from build123d import *

# Parameters (mm, degrees)
BOSS_EXTRUDE1_DEPTH = 11
SKETCH3_W           = 22
SKETCH3_H           = 3
BOSS_EXTRUDE2_DEPTH = 10.2
BOSS_EXTRUDE3_DEPTH = 5
SKETCH5_R           = 1.035
SKETCH5_R_2         = 1.1
CUT_EXTRUDE1_DEPTH  = 34.004922045
SKETCH6_W           = 7
SKETCH6_H           = 7
BOSS_EXTRUDE4_DEPTH = 5
SKETCH7_R           = 1.65
CUT_EXTRUDE2_DEPTH  = 29.50349942
FILLET1_R           = 1


with BuildPart() as part:
    # Sketch1 → Boss-Extrude1 (new, symmetric)
    with BuildSketch(Plane(origin=(0, 0, 0), x_dir=(0, 0, -1), z_dir=(1, 0, 0))):
        Polygon((-13.0089, 0), (13.0089, 0), (13.0089, 3), (5.7589, 3), (5.7589, 1.5), (-5.7589, 1.5), (-5.7589, 3), (-13.0089, 3), align=None)
    extrude(amount=BOSS_EXTRUDE1_DEPTH, both=True)

    # Sketch3 → Boss-Extrude2 (add)
    with BuildSketch(Plane.XZ):
        with Locations((0, -14.5089)):
            Rectangle(SKETCH3_W, SKETCH3_H)
        with Locations((0, 14.5089)):
            Rectangle(SKETCH3_W, SKETCH3_H)
    extrude(amount=-BOSS_EXTRUDE2_DEPTH)

    # Sketch4 → Boss-Extrude3 (add)
    with BuildSketch(Plane(origin=(11, 0, 0), x_dir=(0, 0, -1), z_dir=(1, 0, 0))):
        with BuildLine():
            Line((-8.8, 10.2), (-16.0089, 10.2))
            Line((-16.0089, 10.2), (-16.0089, 0))
            Line((-16.0089, 0), (16.0089, 0))
            Line((16.0089, 0), (16.0089, 10.2))
            Line((16.0089, 10.2), (8.8, 10.2))
            ThreePointArc((8.8, 10.2), (0, 1.4), (-8.8, 10.2))
        make_face()
    extrude(amount=BOSS_EXTRUDE3_DEPTH)

    # Sketch5 → Cut-Extrude1 (cut, through all)
    with BuildSketch(Plane(origin=(16, 0, 0), x_dir=(0, 0, -1), z_dir=(1, 0, 0))):
        with Locations((-10.5, 5.5)):
            Circle(SKETCH5_R)
        with Locations((10.5, 5.5)):
            Circle(SKETCH5_R)
        with Locations((-8.0089, 2.5)):
            Circle(SKETCH5_R_2)
        with Locations(Location((8.0089, 2.5, 0), (0, 0, 27.035691789))):
            Circle(SKETCH5_R_2)
    extrude(amount=-CUT_EXTRUDE1_DEPTH, mode=Mode.SUBTRACT)

    # Sketch6 → Boss-Extrude4 (add)
    with BuildSketch(Plane.XZ):
        with Locations((0, 19.5089)):
            Rectangle(SKETCH6_W, SKETCH6_H)
        with Locations((12.5, -19.5089)):
            Rectangle(SKETCH6_W, SKETCH6_H)
    extrude(amount=-BOSS_EXTRUDE4_DEPTH)

    # Sketch7 → Cut-Extrude2 (cut, through all)
    with BuildSketch(Plane(origin=(0, 5, 0), x_dir=(1, 0, 0), z_dir=(0, 1, 0))):
        with Locations(Location((0, -19.5089, 0), (0, 0, 270))):
            Circle(SKETCH7_R)
        with Locations(Location((12.5, 19.5089, 0), (0, 0, 270))):
            Circle(SKETCH7_R)
    extrude(amount=-CUT_EXTRUDE2_DEPTH, mode=Mode.SUBTRACT)

    # Fillet1
    fillet1_edges = [part.edges().sort_by_distance(p)[0] for p in [
        (0, 5, 23.0089),
        (12.5, 5, -23.0089),
        (0, 3, 5.7589),
        (0, 3, -5.7589),
        (2.5, 10.2, -16.0089),
        (2.5, 10.2, 16.0089),
    ]]
    fillet(fillet1_edges, radius=FILLET1_R)


solid = part.part
For this review, take the finished solid that the model builds, in its own axes (mm). A direction names the side the tool comes from. Give positions to 0.01 mm unless a question says otherwise; leave off trailing zeros. Order: outer loops, then holes, each group sorted by start corner. A loop starts at its lowest first (then second) coordinate and runs counter-clockwise, first axis right, second up. Notation, with made-up numbers: M 13.25,-21 L 17.25,-21 A9 ccw 17.25,-16 Z; hole C 26,-31.75 d10. An arc over 180 degrees is marked long. Answer in a Markdown table with one row per item. Add a question column.
(1) Consider section C-C on z = -10.5. State the section outline as (x, y) points (3 decimals), and give its area (3 significant figures).
(2) Consider section B-B on y = 2.5. State the section outline as (x, z) points, and give its area (3 significant figures).
(3) For faces 4 (the face through (0, 3, 11)), 5 (the face through (-3.5, 2, 19)), 6 (the face through (9, 2, -20)), list the 3-axis set-ups (+Z, -Z, +X, -X, +Y, -Y) from which the entire face can be reached by the end or side of a thin tool; tool diameter is ignored.
(4) Wall thickness on probe 1 along Z at (x, y) = (0.75, 7.5); probe 2 along Z at (x, y) = (13.25, 3.75); probe 3 along Y at (x, z) = (-6.25, -9.5): over which ranges is each line inside the solid? List them lowest first. Write a range as [from, to].
(5) Mouldability with a two-part tool opening along Y and no side actions: class faces 1 (the face through (0, 5, 17.7)), 2 (the face through (3.5, 2, 19)), 3 (the face through (13.535, 5.546, 11.534)) as +Y half, -Y half, draft (parallel to the pull), parting line (faces both ways), or undercut.
(6) For pin 1 (2 mm diameter, centred on x = 0.5, z = 11.5, fed in from +Y); pin 2 (3 mm diameter, centred on x = 0.5, z = 19.5, fed in from +Y); pin 3 (3.5 mm diameter, centred on x = -4.5, y = 5, fed in from -Z), all flat-tipped, find the tip position at first contact; note any pin that passes through.
(7) Consider section D-D on x = 0. State the section outline as (y, z) points, and give its area (3 significant figures).
(8) Consider section A-A on x = 11.75. State the section outline as (y, z) points (3 decimals), and give its area (3 significant figures).
Evaluation:
| question | item | result |
|---|---|---|
| 1 | outline | M -11,0 L 16,0 L 16,4.465 L 11,4.465 L 11,3 L -11,3 Z; M 11,6.535 L 16,6.535 L 16,10.2 L 11,10.2 Z |
| 1 | area | 107 mm^2 |
| 2 | outline | M -11,-16.01 L 9,-16.01 L 9,-23.01 L 16,-23.01 L 16,-9.11 L -11,-9.11 Z; M -11,-6.91 L 16,-6.91 L 16,-4.26 L 11,-4.26 L 11,-5.89 L -11,-5.89 Z; M -11,5.89 L 11,5.89 L 11,4.26 L 16,4.26 L 16,6.91 L -11,6.91 Z; M -11,9.11 L 16,9.11 L 16,16.01 L 3.5,16.01 L 3.5,23.01 L -3.5,23.01 L -3.5,16.01 L -11,16.01 Z; hole C 0,19.51 d3.3; hole C 12.5,-19.51 d3.3 |
| 2 | area | 525 mm^2 |
| 3 | face 4 | -X, +Y |
| 3 | face 5 | +Z, -X, +Y, -Y |
| 3 | face 6 | -Z, -X, +Y, -Y |
| 4 | probe 1 | z = [-16.01, -13.01], [13.01, 16.01] |
| 4 | probe 2 | z = [-23.01, -20.98], [-18.04, -5.99], [5.99, 16.01] |
| 4 | probe 3 | y = [0, 3] |
| 5 | face 1 | +Y half |
| 5 | face 2 | draft |
| 5 | face 3 | undercut |
| 6 | pin 1 | stops at y = 3 |
| 6 | pin 2 | stops at y = 5 |
| 6 | pin 3 | stops at z = -16.01 |
| 7 | outline | M 0,-16.01 L 9.2,-16.01 A1 ccw 10.2,-15.01 L 10.2,-13.01 L 3,-13.01 L 3,-8.99 A1.1 cw long 3,-7.03 L 3,-6.76 A1 ccw 2,-5.76 L 1.5,-5.76 L 1.5,5.76 L 2,5.76 A1 ccw 3,6.76 L 3,7.03 A1.1 cw long 3,8.99 L 3,13.01 L 10.2,13.01 L 10.2,15.01 A1 ccw 9.2,16.01 L 5,16.01 L 5,17.86 L 0,17.86 Z; M 0,21.16 L 5,21.16 L 5,22.01 A1 ccw 4,23.01 L 0,23.01 Z |
| 7 | area | 133 mm^2 |
| 8 | outline | M 0,-23.009 L 4,-23.009 A1 ccw 5,-22.009 L 5,-20.979 L 0,-20.979 Z; M 0,-18.039 L 5,-18.039 L 5,-16.009 L 9.2,-16.009 A1 ccw 10.2,-15.009 L 10.2,-8.8 A8.8 cw 10.2,8.8 L 10.2,15.009 A1 ccw 9.2,16.009 L 0,16.009 Z; hole C 2.5,-8.009 d2.2; hole C 2.5,8.009 d2.2; hole C 5.5,-10.5 d2.07; hole C 5.5,10.5 d2.07 |
| 8 | area | 210 mm^2 |
